Source: CAD feature listing. Evaluate the final solid. Frame: model axes, mm. A direction names the side the tool comes from. Round coordinates to 2 decimals unless told otherwise and drop trailing zeros. Loops run counter-clockwise (first coordinate to the right, second up) from the corner with the lowest first, then second, coordinate; pieces in that order, holes last. Notation, with made-up numbers: (-4.75, 24) - (5.25, 24) arc R28 cw to (5.25, 51) - close; hole circle Ø7 at (77.25, -33.75). An arc over 180 degrees is marked (long way). One line per question, with ' | ' between items.
from build123d import *

# Parameters (mm, degrees)
SKETCH1_W           = 55
SKETCH1_H           = 40
SKETCH1_R           = 1.4
BOSS_EXTRUDE1_DEPTH = 1.5
SKETCH2_W           = 9.907742448
SKETCH2_H           = 22.517169438
SKETCH2_W_2         = 6.62013717
SKETCH2_H_2         = 10.343964327
BOSS_EXTRUDE2_DEPTH = 20


with BuildPart() as part:
    # Sketch1 → Boss-Extrude1 (new body)
    with BuildSketch(Plane(origin=(0, 0, 0), x_dir=(1, 0, 0), z_dir=(0, 1, 0))):
        Rectangle(SKETCH1_W, SKETCH1_H)
        with Locations(Location((-24.09, 17.06, 0), (0, 0, 270))):
            Circle(SKETCH1_R, mode=Mode.SUBTRACT)
        with Locations(Location((-24.09, -16.59, 0), (0, 0, 270))):
            Circle(SKETCH1_R, mode=Mode.SUBTRACT)
        with Locations(Location((24.56, -16.59, 0), (0, 0, 270))):
            Circle(SKETCH1_R, mode=Mode.SUBTRACT)
        with Locations(Location((24.56, 17.06, 0), (0, 0, 270))):
            Circle(SKETCH1_R, mode=Mode.SUBTRACT)
    extrude(amount=BOSS_EXTRUDE1_DEPTH)

    # Sketch2 → Boss-Extrude2 (add)
    with BuildSketch(Plane(origin=(0, 1.5, 0), x_dir=(1, 0, 0), z_dir=(0, 1, 0))):
        with Locations((11.877828391, 3.030915981)):
            Rectangle(SKETCH2_W, SKETCH2_H)
        Polygon((5.930539548, 16.964101497), (-17.184772736, 16.964101497), (-17.184772736, 3.668659348), (-12.771347956, 3.668659348), (-12.771347956, -15.309067205), (1.07577229, -15.309067205), (1.07577229, -1.351611339), (5.930539548, -1.351611339), align=None)
        with Locations((-22.149875613, -5.171982164)):
            Rectangle(SKETCH2_W_2, SKETCH2_H_2)
    extrude(amount=BOSS_EXTRUDE2_DEPTH)


solid = part.part
1. Access query for faces 1 (the flat face through (6.924, 11, -3)), 2 (the flat face through (12, 11, -14.29)), 3 (the flat face through (3, 11, 1.352)), 4 (the flat face through (-22, 11, 0)), 5 (the flat face through (-15, 11, -3.669)). Directions: +Z, -Z, +X, -X, +Y, -Y. A direction counts if a zero-diameter tool reaches every point of the face in a straight line with its end or side. Return the directions, or none.
Worked out:
face 1: +Z, -Z, +Y | face 2: -Z, +X, +Y | face 3: +Z, +Y | face 4: -Z, -X, +Y | face 5: +Z, -X, +Y
2. Contact query for flat-ended pins moving along their axis: P1, Ø8, axis at x = -2, y = 17.5, coming from the -Z side; P2, Ø10, axis at y = 12.5, z = -1, coming from the +X side; P3, Ø1.5, axis at y = 4.5, z = -2, coming from the -X side. Output: stop coordinate, or through.
Worked out:
P1: stops at z = -16.96 | P2: stops at x = 16.83 | P3: stops at x = -12.77
3. Section query D-D, the plane z = -7. Return loops of the section in (x, y).
Worked out:
outline: (-27.5, 0) - (27.5, 0) - (27.5, 1.5) - (16.83, 1.5) - (16.83, 21.5) - (6.92, 21.5) - (6.92, 1.5) - (5.93, 1.5) - (5.93, 21.5) - (-17.18, 21.5) - (-17.18, 1.5) - (-27.5, 1.5) - close
4. Material intervals for probe 1 along X at (y, z) = (0.6, 16.59); probe 2 along X at (y, z) = (13.25, 1); probe 3 along X at (y, z) = (15.5, -2.5), sorted ascending.
Worked out:
probe 1: x = -27.5 to -25.49, -22.69 to 23.16, 25.96 to 27.5 | probe 2: x = -25.46 to -18.84, -12.77 to 5.93, 6.92 to 16.83 | probe 3: x = -12.77 to 5.93, 6.92 to 16.83
5. Mould query, pull axis X, two halves, no side actions, for faces 6 (the flat face through (-12.771, 11, 6)), 7 (the flat face through (16.832, 11, -3)), 8 (the flat face through (-6, 11, 15.309)), 9 (the flat face through (-25.46, 11, 5)). Classes: released by +X, released by -X, zero draft, split by the parting line, or undercut.
Worked out:
face 6: undercut | face 7: released by +X | face 8: zero draft | face 9: released by -X
6. Section query A-A, the plane x = 24.56. Return loops of the section in (y, z).
Worked out:
outline: (0, -20) - (1.5, -20) - (1.5, -18.46) - (0, -18.46) - close; (0, -15.66) - (1.5, -15.66) - (1.5, 15.19) - (0, 15.19) - close; (0, 17.99) - (1.5, 17.99) - (1.5, 20) - (0, 20) - close
7. Section query B-B, the plane z = 16.59. Return loops of the section in (x, y).
Worked out:
outline: (-27.5, 0) - (-25.49, 0) - (-25.49, 1.5) - (-27.5, 1.5) - close; (-22.69, 0) - (23.16, 0) - (23.16, 1.5) - (-22.69, 1.5) - close; (25.96, 0) - (27.5, 0) - (27.5, 1.5) - (25.96, 1.5) - close
8. Section query C-C, the plane y = 3.5. Return loops of the section in (x, z).
Worked out:
outline: (-25.46, 0) - (-18.84, 0) - (-18.84, 10.34) - (-25.46, 10.34) - close; (-17.18, -16.96) - (5.93, -16.96) - (5.93, 1.35) - (1.08, 1.35) - (1.08, 15.31) - (-12.77, 15.31) - (-12.77, -3.67) - (-17.18, -3.67) - close; (6.92, -14.29) - (16.83, -14.29) - (16.83, 8.23) - (6.92, 8.23) - close
